Build history of the part. All positions in model axes, mm. A direction names the side the tool comes from. Give positions to 0.01 mm unless a question says otherwise; leave off trailing zeros. Order: outer loops, then holes, each group sorted by start corner. A loop starts at its lowest first (then second) coordinate and runs counter-clockwise, first axis right, second up. Notation, with made-up numbers: M 26.5,72 L 79.5,72 A29 cw 79.5,103 Z; hole C 18.5,71 d8. An arc over 180 degrees is marked long. Answer as CSV lines item,"result".
from build123d import *

# Parameters (mm, degrees)
SKETCH1_W           = 19
SKETCH1_H           = 6.5
BOSS_EXTRUDE1_DEPTH = 50
SKETCH2_W           = 19
SKETCH2_H           = 58
BOSS_EXTRUDE2_DEPTH = 3.7
CUT_EXTRUDE1_DEPTH  = 54.937950462


with BuildPart() as part:
    # Sketch1 → Boss-Extrude1 (new body)
    with BuildSketch(Plane.XY):
        Rectangle(SKETCH1_W, SKETCH1_H)
    extrude(amount=BOSS_EXTRUDE1_DEPTH)

    # Sketch2 → Boss-Extrude2 (add)
    with BuildSketch(Plane(origin=(0, 3.25, 0), x_dir=(1, 0, 0), z_dir=(0, 1, 0))):
        with Locations((0, -21)):
            Rectangle(SKETCH2_W, SKETCH2_H)
    extrude(amount=BOSS_EXTRUDE2_DEPTH)

    # Sketch3 → Cut-Extrude1 (cut, through all)
    with BuildSketch(Plane.ZY.offset(9.5)):
        Polygon((50, 4.75), (50, -3.25), (5, -3.25), (5, 0.75), align=None)
    extrude(amount=-CUT_EXTRUDE1_DEPTH, mode=Mode.SUBTRACT)


solid = part.part
Item 1: 3-axis set-ups, long thin cutter, end or side, ignore diameter. For faces 1 (the flat face through (0, 0, 0)), 2 (the flat face through (0, -1, 5)), 3 (the flat face through (0, -3.25, 2)): which of +Z, -Z, +X, -X, +Y, -Y reach the whole face in a straight line?
Geometry says:
face 1,"-Z, +X, -X, -Y"
face 2,"+Z, +X, -X, -Y"
face 3,"+Z, -Z, +X, -X, -Y"
Item 2: Band-saw the part on C-C (y = 4.25). Give the cut face in (x, z) (3 decimals).
Geometry says:
outline,"M -9.5,-8 L 9.5,-8 L 9.5,44.375 L -9.5,44.375 Z"
Item 3: Band-saw the part on B-B (z = -1.5). Give the cut face in (x, y).
Geometry says:
outline,"M -9.5,3.25 L 9.5,3.25 L 9.5,6.95 L -9.5,6.95 Z"
Item 4: Band-saw the part on A-A (x = -5.5). Give the cut face in (y, z), and give its area (3 significant figures).
Geometry says:
outline,"M -3.25,0 L 3.25,0 L 3.25,-8 L 6.95,-8 L 6.95,50 L 4.75,50 L 0.75,5 L -3.25,5 Z"
area,"270 mm2"
Item 5: Probe line 1 along Z through (x, y) = (-3, -1.75); line 2 along Y through (x, z) = (-7.75, -3); line 3 along Y through (x, z) = (7.5, 35.5). List the from-to ranges inside material, lowest first. Write a range as from..to.
Geometry says:
line 1,"z = 0..5"
line 2,"y = 3.25..6.95"
line 3,"y = 3.46..6.95"
Item 6: Drop flat-ended pins along their axis: pin 1 (1.5 mm diameter, centred on x = -0.5, z = 8.5, fed in from -Y); pin 2 (9 mm diameter, centred on x = -1, z = -4, fed in from -Y); pin 3 (4.5 mm diameter, centred on x = -1.5, y = -2, fed in from +Z). Give the stop position or say it passes through.
Geometry says:
pin 1,"stops at y = 0.99"
pin 2,"stops at y = -3.25"
pin 3,"stops at z = 5"
